Input: dimensioned drawing with shaded views. Units: mm. Origin: part minimum x, y, z. A direction names the side the tool comes from. Round coordinates to 2 decimals unless told otherwise and drop trailing zeros. Loops run counter-clockwise (first coordinate to the right, second up) from the corner with the lowest first, then second, coordinate; pieces in that order, holes last. Notation, with made-up numbers: M -2,48.5 L 41,48.5 A8 cw 41,59.5 Z; hole C -36.75,25.5 d2. An arc over 180 degrees is marked long. Put each result on its own line as item: value. Start each with the question number.
1) Line query: probe 1 along X at (y, z) = (5.25, 7); probe 2 along X at (y, z) = (12.75, 5.75); probe 3 along X at (y, z) = (8, 8). Output: solid intervals per line, ascending.
2) Section A-A on z = 7. Output: boundary loops of the cut face in (x, y), plus the area to 4 significant figures.
3) Section D-D on x = 15. Output: boundary loops of the cut face in (y, z).
4) Draft query along Z for the marked faces 3, 4 and 5. Return one class per face: +Z half, -Z half, draft (parallel to the pull), parting line (faces both ways), or undercut.
5) Pin query (flat end, axial travel): pin 1 (1.5 mm diameter, centred on x = 12, y = 7, fed in from +Z); pin 2 (8 mm diameter, centred on x = 12.5, z = 8.5, fed in from +Y); pin 3 (1 mm diameter, centred on x = 6, z = 9, fed in from +Y); pin 4 (1.8 mm diameter, centred on x = 15, z = 7, fed in from +Y). Return the tip coordinate at first contact, or that it passes through.
6) Reachability of the marked faces 1 and 2 from +Z, -Z, +X, -X, +Y, -Y: full face, straight path, thin tool, end or side. Return the list, or none.
7) Section C-C on z = 2.75. Output: boundary loops of the cut face in (x, y), plus the area to 3 significant figures.
8) Section B-B on y = 7. Output: boundary loops of the cut face in (x, z).
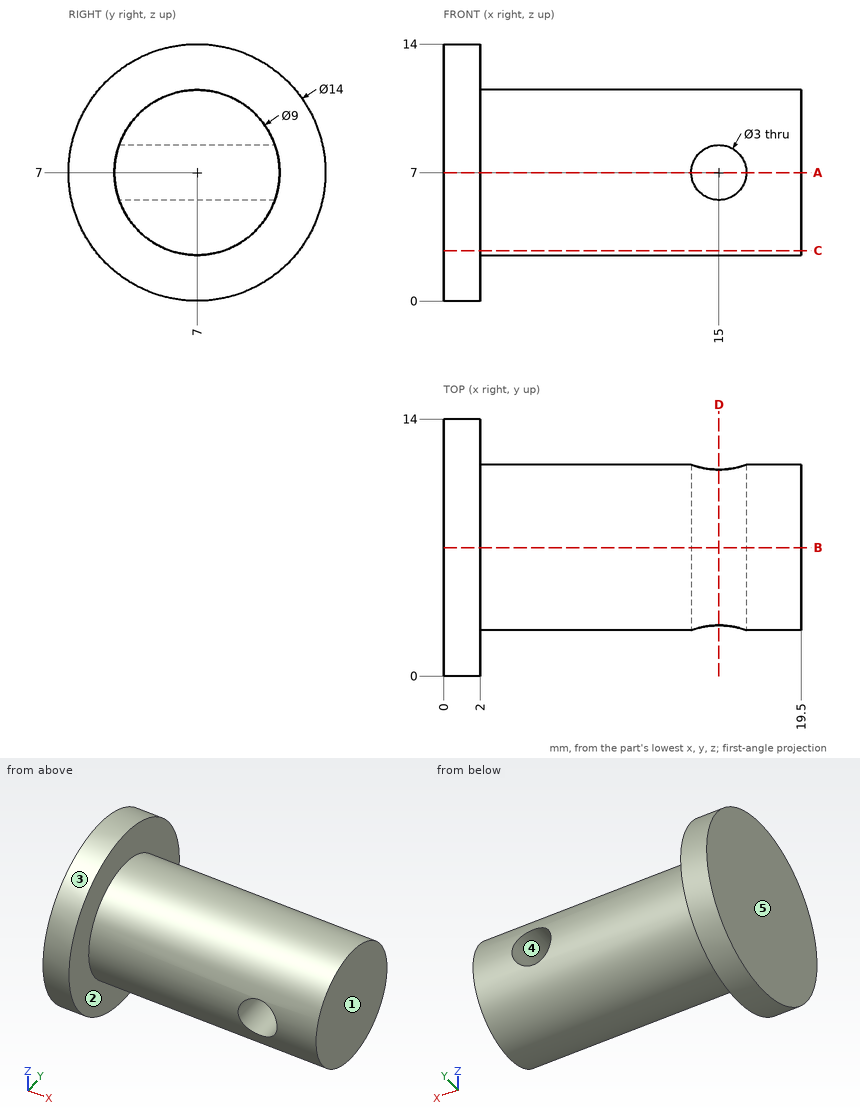
Geometry results:
1. probe 1: x = 0 to 13.5, 16.5 to 19.5
1. probe 2: x = 0 to 2
1. probe 3: x = 0 to 13.88, 16.12 to 19.5
2. outline: M 0,0 L 2,0 L 2,2.5 L 13.5,2.5 L 13.5,11.5 L 2,11.5 L 2,14 L 0,14 Z; M 16.5,2.5 L 19.5,2.5 L 19.5,11.5 L 16.5,11.5 Z
2. area: 158.5 mm²
3. outline: M 2.76,5.5 A4.5 ccw 11.24,5.5 Z; M 2.76,8.5 L 11.24,8.5 A4.5 ccw Z
4. face 3: parting line
4. face 4: undercut
4. face 5: draft
5. pin 1: stops at z = 11.5
5. pin 2: stops at y = 11.5
5. pin 3: stops at y = 11.24
5. pin 4: passes through
6. face 1: +Z, -Z, +X, +Y, -Y
6. face 2: +X
7. outline: M 0,1.44 L 2,1.44 L 2,5.52 L 19.5,5.52 L 19.5,8.48 L 2,8.48 L 2,12.56 L 0,12.56 Z
7. area: 74.0 mm²
8. outline: M 0,0 L 2,0 L 2,2.5 L 19.5,2.5 L 19.5,11.5 L 2,11.5 L 2,14 L 0,14 Z; hole C 15,7 d3
